Geometry: final body of the model. Coordinates: model frame, mm. A direction names the side the tool comes from. Round coordinates to 2 decimals unless told otherwise and drop trailing zeros. Loops run counter-clockwise (first coordinate to the right, second up) from the corner with the lowest first, then second, coordinate; pieces in that order, holes last. Notation, with made-up numbers: M 29.5,-29 L 86.5,-29 A17 cw 86.5,2 Z; hole C -11,-13 d4. An arc over 180 degrees is marked long. Write each question's results on one line, items separated by ' | '.
Autodesk Inventor part; units mm, degrees
ref_plane "YZ Plane" through (0, 0, 0) normal (1, 0, 0) x (0, 1, 0)
ref_plane "XZ Plane" through (0, 0, 0) normal (0, 1, 0) x (-1, 0, 0)
ref_plane "XY Plane" through (0, 0, 0) normal (0, 0, 1) x (1, 0, 0)
sketch "Sketch1" plane through (0, 0, 0) normal (0, 1, 0) x (-1, 0, 0)
  line L0 (0.53, 20.25) -> (-28.77, 20.25)
  line L1 (-28.77, 20.25) -> (-28.77, -20.25)
  line L2 (-28.77, -20.25) -> (0.53, -20.25)
  line L3 (0.53, -20.25) -> (0.53, 20.25)
  point P0 (0, 0)
  dimension "d0" = 40.5
  dimension "d1" = 29.3
  dimension "d2" = -0.53
  dimension "d3" = 20.25
extrude "Plate1" add sketch "Sketch1" along normal blind 1.5
sketch "Sketch2" plane through (28.77, 0, 21.75) normal (0, 0, -1) x (-1, 0, 0)
  line L0 (29.3, 0) -> (0, 0)
  line L1 (0, 0) -> (0, 28.14)
  line L2 (0, 28.14) -> (29.3, 28.14)
  line L3 (29.3, 28.14) -> (29.3, 0)
edge flange "Flange1" height 28.14 angle 90 thickness 1.5 bend radius 0.31 thickness toward (0, 0, -1) relief tear relief width 1.5 relief depth 0.75 corner gap 0.31 corner form 0 edges at (14.12, 1.5, 20.25) (14.12, 1.5, -20.25) wall of the first edge with corners at (-0.53, 0, 21.75) (28.77, 0, 21.75) (28.77, 28.14, 21.75) (-0.53, 28.14, 21.75)
bend "Bend1"
corner "Corner1"
sketch "Sketch6" plane through (-0.53, 28.14, 21.75) normal (0, 0, 1) x (1, 0, 0)
  point P0 (0.53, -28.14)
sketch "Sketch8" plane through (28.77, 28.14, -21.75) normal (0, 0, -1) x (-1, 0, 0)
  circle A0 centre (2.5, -2.545) radius 0.7835
  circle A1 centre (2.5, -17.595) radius 0.7835
  circle A2 centre (17.6, -2.545) radius 0.7835
  circle A3 centre (17.6, -17.595) radius 0.7835
  circle A4 centre (37.6, -2.545) radius 0.7835
  circle A5 centre (37.6, -17.595) radius 0.7835
  point P0 (28.77, -28.14)
hole "Hole4" at (26.27, 25.595, -21.75) at (26.27, 10.545, -21.75) at (11.17, 25.595, -21.75) at (11.17, 10.545, -21.75) at (-8.83, 25.595, -21.75) at (-8.83, 10.545, -21.75) direction (0, 0, 1) diameter 2.1 depth 1.5
sketch "Sketch9" plane through (28.77, 28.14, -21.75) normal (0, 0, -1) x (-1, 0, 0)
  circle A0 centre (30.1, -10.07) radius 6
  point P0 (28.77, -28.14)
sketch "Sketch10" plane through (-0.53, 28.14, 21.75) normal (0, 0, 1) x (1, 0, 0)
  point P0 (0.53, -28.14)
sketch "Sketch11" plane through (-0.53, 28.14, 21.75) normal (0, 0, 1) x (1, 0, 0)
  point P0 (0.53, -28.14)
sketch "Sketch15" plane through (0, 0, 0) normal (0, -1, 0) x (1, 0, 0)
  point P0 (0, 0)
sketch "Sketch16" plane through (0, 0, 0) normal (0, -1, 0) x (1, 0, 0)
  circle A0 centre (6.47, 14.94) radius 1.55
  line L0 (28.77, 19.94) -> (-0.53, 19.94)
  line L1 (-0.53, -19.94) -> (-0.53, 19.94)
  circle A1 centre (21.77, 14.94) radius 1.55
  line L2 (28.77, 19.94) -> (28.77, -19.94)
  circle A2 centre (6.47, 4.8) radius 1.55
  circle A3 centre (21.77, 4.8) radius 1.55
  point P0 (0, 0)
  dimension "d65" = 3.1
  dimension "d66" = 5
  dimension "d67" = 7
  dimension "d68" = 3.1
  dimension "d69" = 5
  dimension "d70" = 7
  dimension "d71" = 3.1
  dimension "d72" = 15.14
  dimension "d73" = 7
  dimension "d74" = 3.1
  dimension "d75" = 15.14
  dimension "d76" = 7
extrude "Cut6" cut sketch "Sketch16" against normal blind 1.5
sketch "Sketch18" plane through (-0.53, 28.14, 21.75) normal (0, 0, 1) x (1, 0, 0)
  circle A0 centre (-0.8, -10.07) radius 6
  point P0 (0.53, -28.14)
fillet "Corner Round1" radius 1 4 edges at (-0.53, 28.14, -21) (28.77, 28.14, -21) (28.77, 28.14, 21) (-0.53, 28.14, 21)
sketch "Sketch19" plane through (-0.53, 1.81, 21.75) normal (0, 0, 1) x (1, 0, 0)
  circle A0 centre (6.1, 24.26) radius 0.7835
  circle A1 centre (19.32, 23.26) radius 0.7835
  circle A2 centre (26.62, 16.26) radius 0.7835
  circle A3 centre (19.32, 9.26) radius 0.7835
  circle A4 centre (6.1, 8.26) radius 0.7835
  point P0 (0.53, -1.81)
hole "Hole6" at (5.57, 26.07, 21.75) at (18.79, 25.07, 21.75) at (26.09, 18.07, 21.75) at (18.79, 11.07, 21.75) at (5.57, 10.07, 21.75) direction (0, 0, -1) diameter 2.1 depth 1.5
hole "Hole7" at (-1.33, 18.07, 21.75) direction (0, 0, -1) diameter 13.5 depth 1.5
hole "Hole8" at (-1.33, 18.07, -21.75) direction (0, 0, 1) diameter 13.5 depth 1.5
sketch "Sketch20" plane through (-0.53, 1.81, 21.75) normal (0, 0, 1) x (1, 0, 0)
  arc A0 (0, 9.5576) -> (0, 22.9624) centre (-0.8, 16.26) ccw
  line L0 (3.973, 11.487) -> (18.8159, 26.33)
  line L1 (1, 26.33) -> (28.3, 26.33)
  arc A1 (1, 26.33) -> (0, 25.33) centre (1, 25.33) ccw
  line L2 (0, 22.9624) -> (0, 25.33)
  line L3 (18.8159, 26.33) -> (1, 26.33)
  arc A2 (1, 26.33) -> (0, 25.33) centre (1, 25.33) ccw
  line L4 (0, 25.33) -> (0, 22.9624)
  arc A3 (3.973, 11.487) -> (0, 22.9624) centre (-0.8, 16.26) ccw
  point P0 (0.53, -1.81)
  dimension "d110" = 45
  dimension "d111" = 0
extrude "Cut8" cut sketch "Sketch20" against normal blind 1.5
mirror "Mirror1" about plane through (0, 0, 0) normal (0, 0, 1) of "Cut8"
equation "\"d55\" = Thickness"
equation "\"d77\" = Thickness"
equation "\"d94\" = Thickness"
equation "\"d101\" = Thickness"
equation "\"d108\" = Thickness"
equation "\"d112\" = Thickness"
equation "\"d4\" = Thickness"
equation "\"d5\" = BendReliefWidth"
equation "\"d6\" = BendReliefDepth"
equation "\"d7\" = MinimumRemnant"
equation "\"d8\" = TransitionRadius"
equation "\"d11\" = BendRadius"
equation "\"d12\" = CornerReliefSize"
equation "\"d13\" = GapSize"
equation "\"d14\" = JacobiRadiusSize"
equation "\"BendReliefWidth\" = Thickness"
equation "\"BendReliefDepth\" = 0.5 * Thickness"
equation "\"CornerReliefSize\" = 4 * Thickness"
equation "\"MinimumRemnant\" = 2 * Thickness"
equation "\"TransitionRadius\" = BendRadius"
equation "\"JacobiRadiusSize\" = BendRadius"
equation "\"GapSize\" = Thickness"
properties part number "axis_25_bottom_frame" material "Aluminum 6061-AHC"
1. Ray query, probe 1 along Z at (x, y) = (12, 1.75); probe 2 along Z at (x, y) = (17.75, 13.25); probe 3 along Y at (x, z) = (26.27, -20.65) (3 decimals). Return the intervals inside material, ascending.
Answer key:
probe 1: z = -21.75 to -20.24, 20.24 to 21.75 | probe 2: z = -21.75 to -20.25, 20.25 to 21.75 | probe 3: y = 0.145 to 9.495, 11.595 to 24.545, 26.645 to 28.14
2. Section D-D (x = 11.17). Output: boundary loops of the cut face in (y, z) (3 decimals), then the cut area to 3 significant figures.
Answer key:
outline: M 0,-19.94 A1.81 ccw 1.81,-21.75 L 9.495,-21.75 L 9.495,-20.25 L 1.81,-20.25 A0.31 cw 1.5,-19.94 L 1.5,19.94 A0.31 cw 1.81,20.25 L 21.024,20.25 L 21.024,21.75 L 1.81,21.75 A1.81 ccw 0,19.94 Z; M 11.595,-21.75 L 21.024,-21.75 L 21.024,-20.25 L 11.595,-20.25 Z | area: 119 mm²
3. Section C-C (y = 2.75). Output: boundary loops of the cut face in (x, z), then the cut area to 3 significant figures.
Answer key:
outline: M -0.53,-21.75 L 28.77,-21.75 L 28.77,-20.25 L -0.53,-20.25 Z; M -0.53,20.25 L 28.77,20.25 L 28.77,21.75 L -0.53,21.75 Z | area: 87.9 mm²
4. Draft query along X for faces 1 (the face through (25.05, 18.21, 20.99)), 2 (the face through (1.647, 12.012, 20.99)), 3 (the face through (23, 28.14, -21)). Return one class per face: pulls with the +X half, pulls with the -X half, needs draft (parallel to the pull), parting line crosses it, or undercut.
Answer key:
face 1: undercut | face 2: pulls with the -X half | face 3: needs draft
5. Pin query (flat end, axial travel): P1, Ø8, axis at x = 13.5, z = -3.5, coming from the +Y side; P2, Ø1.3, axis at x = 5.57, y = 10.07, coming from the +Z side; P3, Ø1.3, axis at x = 11.17, y = 10.545, coming from the -Z side. Return the tip coordinate at first contact, or that it passes through.
Answer key:
P1: stops at y = 1.5 | P2: stops at z = -20.25 | P3: stops at z = 20.25
6. Section A-A (z = 4.8). Output: boundary loops of the cut face in (x, y), then the cut area to 4 significant figures.
Answer key:
outline: M -0.53,0 L 4.92,0 L 4.92,1.5 L -0.53,1.5 Z; M 8.02,0 L 20.22,0 L 20.22,1.5 L 8.02,1.5 Z; M 23.32,0 L 28.77,0 L 28.77,1.5 L 23.32,1.5 Z | area: 34.65 mm²
7. Access query for faces 4 (the face through (14, 1.5, 0)), 5 (the face through (14, 0, 0)), 6 (the face through (10.46, 9.77, -20.99)), 7 (the face through (17.75, 25.21, 20.99)). Directions: +Z, -Z, +X, -X, +Y, -Y. A direction counts if a zero-diameter tool reaches every point of the face in a straight line with its end or side. Return the directions, or none.
Answer key:
face 4: +X, -X, +Y | face 5: +Z, -Z, +X, -X, -Y | face 6: -Z | face 7: +Z
8. Section B-B (x = 21.77). Output: boundary loops of the cut face in (y, z).
Answer key:
outline: M 0,-19.94 A1.81 ccw 1.81,-21.75 L 28.14,-21.75 L 28.14,-20.25 L 1.81,-20.25 A0.31 cw 1.5,-19.94 L 1.5,3.25 L 0,3.25 Z; M 0,6.35 L 1.5,6.35 L 1.5,13.39 L 0,13.39 Z; M 0,16.49 L 1.5,16.49 L 1.5,19.94 A0.31 cw 1.81,20.25 L 28.14,20.25 L 28.14,21.75 L 1.81,21.75 A1.81 ccw 0,19.94 Z
